```python
from build123d import *

# Parameters (mm, degrees)
SKETCH1_R                = 16
SKETCH1_R_2              = 7.5
SKETCH1_R_3              = 1.5
BOSS_EXTRUDE1_DEPTH      = 27.5
SKETCH2_R                = 9
SKETCH2_R_2              = 7.5
BOSS_EXTRUDE2_DEPTH      = 2
BOSS_EXTRUDE2_DEPTH_BACK = 29.5
SCALE1_SCALE             = 2


with BuildPart() as part:
    # Sketch1 → Boss-Extrude1 (new body)
    with BuildSketch(Plane.XY):
        Circle(SKETCH1_R)
        Circle(SKETCH1_R_2, mode=Mode.SUBTRACT)
        with Locations((-8.485281374, 8.485281374)):
            Circle(SKETCH1_R_3, mode=Mode.SUBTRACT)
        with Locations((8.485281374, 8.485281374)):
            Circle(SKETCH1_R_3, mode=Mode.SUBTRACT)
        with Locations((8.485281374, -8.485281374)):
            Circle(SKETCH1_R_3, mode=Mode.SUBTRACT)
        with Locations((-8.485281374, -8.485281374)):
            Circle(SKETCH1_R_3, mode=Mode.SUBTRACT)
    extrude(amount=BOSS_EXTRUDE1_DEPTH)

    # Sketch2 → Boss-Extrude2 (add, two sides)
    with BuildSketch(Plane.XY.offset(27.5)) as boss_extrude2_sk:
        Circle(SKETCH2_R)
        Circle(SKETCH2_R_2, mode=Mode.SUBTRACT)
    extrude(amount=BOSS_EXTRUDE2_DEPTH)
    extrude(boss_extrude2_sk.sketch, amount=-BOSS_EXTRUDE2_DEPTH_BACK)


with BuildPart() as part_1:
    # Scale1: scaled about (0, 0, 13.75)
    add(part.part.scale(SCALE1_SCALE).moved(Location((0, 0, -13.75))))


solid = part_1.part
```
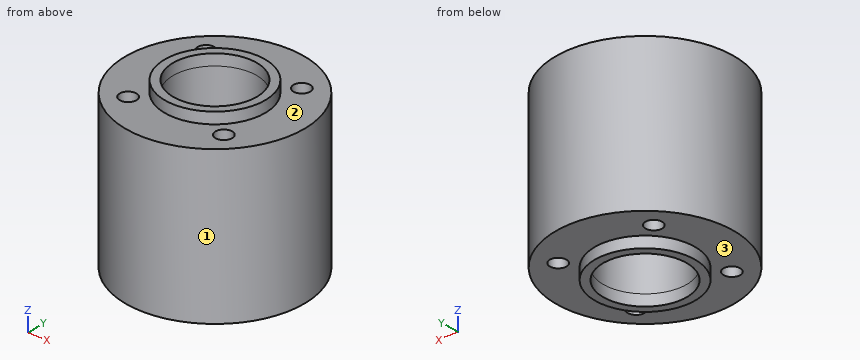
Can you work these out from the model? Positions are in its coordinate system, mm. Face numbers are marked on the shaded views. A direction names the side the tool comes from. Coordinates: 2 decimals unless noted, no trailing zeros. Loops run counter-clockwise (first coordinate to the right, second up) from the corner with the lowest first, then second, coordinate; pieces in that order, holes last. Notation, with made-up numbers: (58, 5.25) -> (84, 5.25) arc R6 cw to (84, 10.25) -> close; hole circle Ø3 at (39, 10.25). An arc over 180 degrees is marked (long way). Put each result on its own line as item: value. Start each with the question number.
Q1. If I drill on line 1 (Y direction, x = 0, z = 42.25); line 2 (Z direction, x = 17, y = -6); line 3 (Y direction, x = -7, z = 16.5), over which ranges is the centre line in solid material (lowest first)? Write a range as [from, to].
Q2. For the marked faces 1, 2 and 3, which set-ups out of +Z, -Z, +X, -X, +Y, -Y let a thin tool reach every point of the face, with its end or its side?
Q3. I'm going to push flat-ended pins straight in: P1, Ø2, axis at x = -2.5, z = 28, coming from the -Y side; P2, Ø1, axis at x = 25, z = 15, coming from the +Y side; P3, Ø2, axis at x = 15, y = 12, coming from the +Z side. Where does each tip first touch, or does it pass through?
Q4. I want a section at C-C (y = 19). Write out the boundary of the cut face in (x, z), plus the area to 3 significant figures.
Q5. I want a section at A-A (y = 0). Write out the boundary of the cut face in (x, z).
Q6. I want a section at D-D (z = 3). Write out the boundary of the cut face in (x, y).
Taken from the geometry:
1. line 1: y = [-18, -15], [15, 18]
1. line 2: z = [-13.75, 41.25]
1. line 3: y = [-31.22, -13.27], [13.27, 31.22]
2. face 1: +Z, -Z
2. face 2: +Z
2. face 3: -Z
3. P1: stops at y = -31.96
3. P2: stops at y = 20.59
3. P3: stops at z = 41.25
4. outline: (-25.75, -13.75) -> (-19.18, -13.75) -> (-19.18, 41.25) -> (-25.75, 41.25) -> close; (-14.76, -13.75) -> (14.76, -13.75) -> (14.76, 41.25) -> (-14.76, 41.25) -> close; (19.18, -13.75) -> (25.75, -13.75) -> (25.75, 41.25) -> (19.18, 41.25) -> close
4. area: 2,350 mm2
5. outline: (-32, -13.75) -> (-18, -13.75) -> (-18, -17.75) -> (-15, -17.75) -> (-15, 45.25) -> (-18, 45.25) -> (-18, 41.25) -> (-32, 41.25) -> close; (15, -17.75) -> (18, -17.75) -> (18, -13.75) -> (32, -13.75) -> (32, 41.25) -> (18, 41.25) -> (18, 45.25) -> (15, 45.25) -> close
6. outline: circle Ø64 at (0, 0); hole circle Ø6 at (-16.97, -16.97); hole circle Ø6 at (-16.97, 16.97); hole circle Ø30 at (0, 0); hole circle Ø6 at (16.97, -16.97); hole circle Ø6 at (16.97, 16.97)
